```python
from build123d import *

# Parameters (mm, degrees)
F1_DEPTH = 125
F2_R     = 46.677597
F3_DEPTH = 80
F4_R     = 15


with BuildPart() as f1:
    # F0 (on Top) → F1 (new body, symmetric)
    with BuildSketch(Plane.XY):
        with BuildLine():
            Line((-900, -875), (900, -875))
            Line((900, -875), (900, 875))
            ThreePointArc((900, 875), (0, 1225), (-900, 875))
            Line((-900, 875), (-900, -875))
        make_face()
    extrude(amount=F1_DEPTH, both=True)

    # F2 (on face) → F3 (join)
    with BuildSketch(Plane(origin=(0, 0, -125), x_dir=(1, 0, 0), z_dir=(0, 0, -1))):
        with Locations((-747.428477, -51.44228)):
            Circle(F2_R)
    extrude(amount=F3_DEPTH)

    # F4
    f4_edges = [f1.edges().sort_by_distance(p)[0] for p in [
        (-794.106074, 51.44228, -205),
    ]]
    fillet(f4_edges, radius=F4_R)


solid = f1.part
```
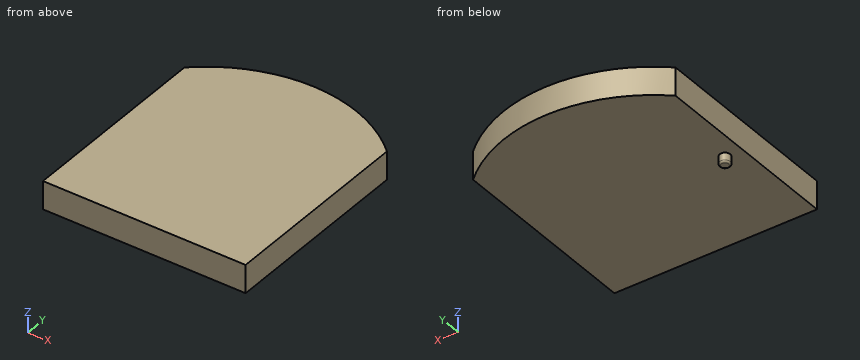
The model under review builds one solid part; all positions refer to its coordinate system, in mm. Round coordinates to 2 decimals unless told otherwise and drop trailing zeros. Loops run counter-clockwise (first coordinate to the right, second up) from the corner with the lowest first, then second, coordinate; pieces in that order, holes last. Notation, with made-up numbers: (62.25, 4.25) -> (74.25, 4.25) arc R35 ccw to (74.25, 39.25) -> close; hole circle Ø10 at (35.5, 27). An arc over 180 degrees is marked (long way). Answer as a JSON object with one key per item and string values. Group by question number.
1) For pin 1 Ø8 at (x, z) = (-704, -104.5) entering from +Y; pin 2 Ø6 at (x, y) = (-549, 254.5) entering from -Z; pin 3 Ø8 at (y, z) = (934.5, -126.5) entering from +X, all flat-tipped, find the tip position at first contact; note any pin that passes through.
2) We need section A-A on z = 35. Write out the cut boundary in (x, y).
3) We need section B-B on x = -171. Write out the cut boundary in (y, z), then the cut area to 3 significant figures.
4) For line 1 (Z direction, x = 176, y = 118.5); line 2 (Y direction, x = 20, z = -104); line 3 (Y direction, x = -12, z = 29), list the stretches that pass through material, from the lowest coordinate up. Write a range as [from, to].
Result set:
{
 "1": {"pin 1": "y = 1026.26", "pin 2": "z = -125", "pin 3": "x = 835.04"},
 "2": {"outline": "(-900, -875) -> (900, -875) -> (900, 875) arc R1332.14 ccw to (-900, 875) -> close"},
 "3": {"outline": "(-875, -125) -> (1213.98, -125) -> (1213.98, 125) -> (-875, 125) -> close", "area": "522,000 mm²"},
 "4": {"line 1": "[-125, 125]", "line 2": "[-875, 1224.85]", "line 3": "[-875, 1224.95]"}
}
